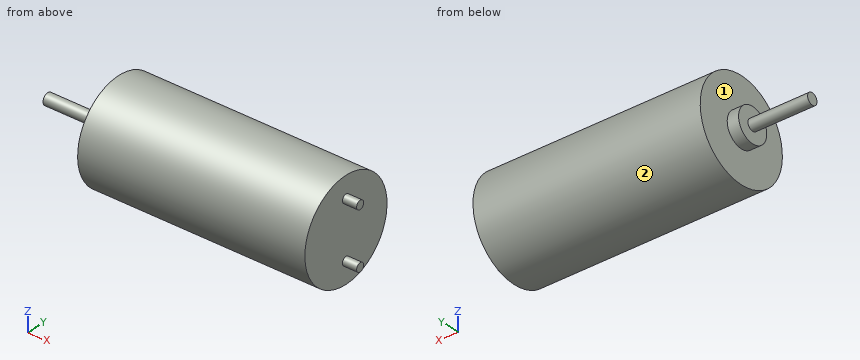
```python
from build123d import *

# Parameters (mm, degrees)
SKETCH1_R           = 3.5
BOSS_EXTRUDE1_DEPTH = 16
SKETCH2_R           = 1.2
BOSS_EXTRUDE2_DEPTH = 0.8
SKETCH3_R           = 0.4
BOSS_EXTRUDE3_DEPTH = 4.2
SKETCH4_R           = 0.3
BOSS_EXTRUDE4_DEPTH = 1


with BuildPart() as part:
    # Sketch1 → Boss-Extrude1 (new body)
    with BuildSketch(Plane(origin=(0, 0, 0), x_dir=(0, 0, -1), z_dir=(1, 0, 0))):
        Circle(SKETCH1_R)
    extrude(amount=BOSS_EXTRUDE1_DEPTH)

    # Sketch2 → Boss-Extrude2 (add)
    with BuildSketch(Plane.ZY):
        Circle(SKETCH2_R)
    extrude(amount=BOSS_EXTRUDE2_DEPTH)

    # Sketch3 → Boss-Extrude3 (add)
    with BuildSketch(Plane.ZY.offset(0.8)):
        Circle(SKETCH3_R)
    extrude(amount=BOSS_EXTRUDE3_DEPTH)

    # Sketch4 → Boss-Extrude4 (add)
    with BuildSketch(Plane(origin=(16, 0, 0), x_dir=(0, 0, -1), z_dir=(1, 0, 0))):
        with Locations((-2, 0)):
            Circle(SKETCH4_R)
        with Locations((2, 0)):
            Circle(SKETCH4_R)
    extrude(amount=BOSS_EXTRUDE4_DEPTH)


solid = part.part
```
For this review, take the finished solid that the model builds, in its own axes (mm). Face numbers are marked on the shaded views. A direction names the side the tool comes from. Round coordinates to 2 decimals unless told otherwise and drop trailing zeros. Order: outer loops, then holes, each group sorted by start corner. A loop starts at its lowest first (then second) coordinate and runs counter-clockwise, first axis right, second up. Notation, with made-up numbers: (35, 48) -> (61, 48) arc R28 cw to (61, 80) -> close; hole circle Ø3 at (83, -3.75). An arc over 180 degrees is marked (long way). Use a Markdown table: item, result.
Item 1: Machinability: for the marked faces 1 and 2, which of the approach directions +Z, -Z, +X, -X, +Y, -Y give a long, thin tool a straight path to every point of the face, cutting with its end or side? Answer none if there is none.
Resolved:
| item | result |
|---|---|
| face 1 | -X |
| face 2 | +X, -X |
Item 2: Take a section at B-B (y = 1). State the section outline as (x, z) points, plus the area to 3 significant figures.
Resolved:
| item | result |
|---|---|
| outline | (-0.8, -0.66) -> (0, -0.66) -> (0, -3.35) -> (16, -3.35) -> (16, 3.35) -> (0, 3.35) -> (0, 0.66) -> (-0.8, 0.66) -> close |
| area | 108 mm² |
Item 3: For line 1 along X through (y, z) = (-2.25, -2); line 2 along X through (y, z) = (-1, -0.25); line 3 along Y through (x, z) = (5, 1.5), list the stretches that pass through material, from the lowest coordinate up. Write a range as [from, to].
Resolved:
| item | result |
|---|---|
| line 1 | x = [0, 16] |
| line 2 | x = [-0.8, 16] |
| line 3 | y = [-3.16, 3.16] |
Item 4: Take a section at D-D (z = -2). State the section outline as (x, y) points.
Resolved:
| item | result |
|---|---|
| outline | (0, -2.87) -> (16, -2.87) -> (16, -0.3) -> (17, -0.3) -> (17, 0.3) -> (16, 0.3) -> (16, 2.87) -> (0, 2.87) -> close |
Item 5: Take a section at C-C (x = 9.25). State the section outline as (y, z) points, plus the area to 3 significant figures.
Resolved:
| item | result |
|---|---|
| outline | circle Ø7 at (0, 0) |
| area | 38.5 mm² |
Item 6: Take a section at A-A (z = 0). State the section outline as (x, y) points.
Resolved:
| item | result |
|---|---|
| outline | (-5, -0.4) -> (-0.8, -0.4) -> (-0.8, -1.2) -> (0, -1.2) -> (0, -3.5) -> (16, -3.5) -> (16, 3.5) -> (0, 3.5) -> (0, 1.2) -> (-0.8, 1.2) -> (-0.8, 0.4) -> (-5, 0.4) -> close |
Item 7: For pin 1 (1 mm diameter, centred on x = 9, y = 1, fed in from -Z); pin 2 (1.5 mm diameter, centred on x = 13.5, z = -2, fed in from +Y); pin 3 (2 mm diameter, centred on y = 2, z = -1.5, fed in from -X), all flat-tipped, find the tip position at first contact; note any pin that passes through.
Resolved:
| item | result |
|---|---|
| pin 1 | stops at z = -3.46 |
| pin 2 | stops at y = 3.27 |
| pin 3 | stops at x = 0 |
